Verification items for the finished model (mm, model axes). A direction names the side the tool comes from. Coordinates: 2 decimals unless noted, no trailing zeros. Order: outer loops, then holes, each group sorted by start corner. A loop starts at its lowest first (then second) coordinate and runs counter-clockwise, first axis right, second up.
Q1. Set-up check for faces 1 (the flat face through (-30, -22, -19)), 2 (the cylindrical face through (-7.493, 13.864, 16.826)), 3 (the flat face through (-2, -22, -22)), 4 (the flat face through (-7, 22, 18)): record each of +Z, -Z, +X, -X, +Y, -Y from which the full face is reachable in a straight line by a thin tool's end or side.
Q2. Cross-section at B-B, the plane x = -32. Record the boundary of the cut face in (y, z), and give its area (4 significant figures).
Q3. Thickness scan on line 1 (Y direction, x = -32, z = -23.65); line 2 (Y direction, x = -7.75, z = 20); line 3 (Z direction, x = -41, y = -19.5). Record the ranges inside material, lowest first.
Q4. Cross-section at D-D, the plane x = -13.5. Record the boundary of the cut face in (y, z).
Q5. Draft check along X on faces 5 (the cylindrical face through (-35.966, -10.909, -23.507)), 6 (the flat face through (-10, 22, -10)), 7 (the cylindrical face through (-8, 0, -18)). Enter one of: pulls with the +X half, pulls with the -X half, needs draft (parallel to the pull), parting line crosses it, or undercut.
Q6. Cross-section at C-C, the plane z = -15. Record the boundary of the cut face in (x, y), and give its area (3 significant figures).
Q7. Cross-section at A-A, the plane y = 11.43. Record the boundary of the cut face in (x, z).
Q8. Depth check by flat-ended pin: P1, Ø4, axis at x = -10, z = 4.5, coming from the +Y side; P2, Ø5.5, axis at x = -3.5, y = 13.5, coming from the +Z side; P3, Ø20.5, axis at y = 28.5, z = 10, coming from the -X side; P4, Ø10.5, axis at x = -32, y = -11.43, coming from the -Z side. Enter the tip coordinate at first touch or a pass-through.
Autodesk Inventor part; units mm, degrees
ref_plane "side_2a_XY" through (-32, -21.925, -19) normal (0, 0, 1) x (1, 0, 0)
ref_plane "side_2a_YZ" through (-32, -21.925, -19) normal (1, 0, 0) x (0, 1, 0)
ref_plane "side_2a_ZX" through (-32, -21.925, -19) normal (0, 1, 0) x (0, 0, 1)
sketch "Skizze_34" plane through (0, 0, 0) normal (0, 1, 0) x (1, 0, 0)
  circle A0 centre (0, 12) radius 10
extrude "Extrusion1" add sketch "Skizze_34" along normal mid plane 2.5
sketch "Skizze_35" plane through (0, 0, 0) normal (0, 1, 0) x (1, 0, 0)
  circle A0 centre (0, 12) radius 6
extrude "Extrusion2" add sketch "Skizze_35" along normal mid plane 85.5
sketch "Skizze_36" plane through (0, -1.3, 0) normal (0, 1, 0) x (1, 0, 0)
  line L0 (-50, 24) -> (-50, 21)
  arc A0 (-50, 21) -> (-48, 19) centre (-48, 21) ccw
  line L1 (-48, 19) -> (-12, 19)
  arc A1 (-10, 17) -> (-12, 19) centre (-12, 17) ccw
  line L2 (-10, 17) -> (-10, 12)
  arc A2 (-10, 12) -> (0, 22) centre (0, 12) ccw
  line L3 (0, 22) -> (-4, 22)
  arc A3 (-5.8856, 23.3333) -> (-4, 22) centre (-4, 24) ccw
  arc A4 (-5.8856, 23.3333) -> (-6.8284, 24) centre (-6.8284, 23) ccw
  line L4 (-6.8284, 24) -> (-50, 24)
  circle A5 centre (0, 12) radius 6
extrude "Extrusion3" add sketch "Skizze_36" against normal blind 41.25
sketch "Skizze_37" plane through (0, 1.3, 0) normal (0, 1, 0) x (1, 0, 0)
  line L0 (-12, -38) -> (-9, -38)
  arc A0 (-9, -38) -> (-7, -36) centre (-9, -36) ccw
  line L1 (-7, -36) -> (-7, 0)
  arc A1 (-5, 2) -> (-7, 0) centre (-5, 0) ccw
  line L2 (-5, 2) -> (0, 2)
  arc A2 (0, 2) -> (-10, 12) centre (0, 12) ccw
  line L3 (-10, 12) -> (-10, 8)
  arc A3 (-11.3333, 6.1144) -> (-10, 8) centre (-12, 8) ccw
  arc A4 (-11.3333, 6.1144) -> (-12, 5.1716) centre (-11, 5.1716) ccw
  line L4 (-12, 5.1716) -> (-12, -38)
  circle A5 centre (0, 12) radius 6
extrude "Extrusion4" add sketch "Skizze_37" along normal blind 41.25
sketch "Sketch5" plane through (-12, 1.3, -5.1716) normal (-1, 0, 0) x (0, 0, 1)
  point P0 (25.1716, 10.13)
hole "Drilling 1" at (-12, 11.43, 20) direction (1, 0, 0) diameter 8 depth 5 countersink diameter 16 countersink angle 90
sketch "Sketch6" plane through (-12, 1.3, -5.1716) normal (-1, 0, 0) x (0, 0, 1)
  point P0 (25.1716, 31.13)
hole "Drilling 2" at (-12, 32.43, 20) direction (1, 0, 0) diameter 8 depth 5 countersink diameter 16 countersink angle 90
sketch "Sketch7" plane through (-48, -1.3, -19) normal (0, 0, 1) x (1, 0, 0)
  point P0 (16, -10.13)
hole "Drilling 3" at (-32, -11.43, -19) direction (0, 0, -1) diameter 8 depth 5 countersink diameter 16 countersink angle 90
sketch "Sketch8" plane through (-48, -1.3, -19) normal (0, 0, 1) x (1, 0, 0)
  point P0 (16, -31.13)
hole "Drilling 4" at (-32, -32.43, -19) direction (0, 0, -1) diameter 8 depth 5 countersink diameter 16 countersink angle 90
ref_plane "side_2a_XY" through (-32, -21.925, -19) normal (0, 0, 1) x (1, 0, 0)
ref_plane "side_2a_YZ" through (-32, -21.925, -19) normal (1, 0, 0) x (0, 1, 0)
ref_plane "side_2a_ZX" through (-32, -21.925, -19) normal (0, 1, 0) x (0, 0, 1)
ref_plane "side_2b_XY" through (-32, -21.925, -24) normal (0, 0, -1) x (1, 0, 0)
ref_plane "side_2b_YZ" through (-32, -21.925, -24) normal (1, 0, 0) x (0, -1, 0)
ref_plane "side_2b_ZX" through (-32, -21.925, -24) normal (0, -1, 0) x (0, 0, -1)
ref_plane "side_1b_XY" through (-7, 21.925, 20) normal (1, 0, 0) x (0, 0, -1)
ref_plane "side_1b_YZ" through (-7, 21.925, 20) normal (0, 0, -1) x (0, 1, 0)
ref_plane "side_1b_ZX" through (-7, 21.925, 20) normal (0, 1, 0) x (1, 0, 0)
ref_plane "side_3b_XY" through (-7, 21.925, 20) normal (1, 0, 0) x (0, 0, -1)
ref_plane "side_3b_YZ" through (-7, 21.925, 20) normal (0, 0, -1) x (0, 1, 0)
ref_plane "side_3b_ZX" through (-7, 21.925, 20) normal (0, 1, 0) x (1, 0, 0)
ref_plane "side_1a_XY" through (-12, 21.925, 20) normal (-1, 0, 0) x (0, 0, -1)
ref_plane "side_1a_YZ" through (-12, 21.925, 20) normal (0, 0, -1) x (0, -1, 0)
ref_plane "side_1a_ZX" through (-12, 21.925, 20) normal (0, -1, 0) x (-1, 0, 0)
ref_plane "side_3a_XY" through (-12, 21.925, 20) normal (-1, 0, 0) x (0, 0, -1)
ref_plane "side_3a_YZ" through (-12, 21.925, 20) normal (0, 0, -1) x (0, -1, 0)
ref_plane "side_3a_ZX" through (-12, 21.925, 20) normal (0, -1, 0) x (-1, 0, 0)
properties part number "MayTec 1.62.842032085_Alu hinges, heavy, type 20 PG 40 (90)"
Check values:
1. face 1: +Z, -X, +Y, -Y
1. face 2: +X, -X
1. face 3: -Z, +X, +Y, -Y
1. face 4: +Z, +X, +Y, -Y
2. outline: (-42.55, -24) - (-36.43, -24) - (-36.43, -23) - (-40.43, -19) - (-42.55, -19) - close; (-28.43, -24) - (-15.43, -24) - (-15.43, -23) - (-19.43, -19) - (-24.43, -19) - (-28.43, -23) - close; (-7.43, -24) - (-1.3, -24) - (-1.3, -19) - (-3.43, -19) - (-7.43, -23) - close
2. area: 94.25 mm2
3. line 1: y = -42.55 to -36.43, -28.43 to -15.43, -7.43 to -1.3
3. line 2: y = 1.3 to 7.43, 15.43 to 28.43, 36.43 to 42.55
3. line 3: z = -24 to -19
4. outline: (-42.55, -24) - (-1.3, -24) - (-1.3, -19) - (-42.55, -19) - close
5. face 5: undercut
5. face 6: pulls with the -X half
5. face 7: parting line crosses it
6. outline: (-10, -42.55) - (-5.2, -42.55) - (-5.2, -42.75) - (5.2, -42.75) - (5.2, -42.55) - (9.54, -42.55) - (9.54, -1.3) - (5.2, -1.3) - (5.2, -1.25) - (9.54, -1.25) - (9.54, 1.25) - (5.2, 1.25) - (5.2, 1.3) - (9.54, 1.3) - (9.54, 42.55) - (5.2, 42.55) - (5.2, 42.75) - (-5.2, 42.75) - (-5.2, 42.55) - (-9.54, 42.55) - (-9.54, 1.3) - (-5.2, 1.3) - (-5.2, 1.25) - (-9.54, 1.25) - (-9.54, -1.25) - (-5.2, -1.25) - (-5.2, -1.3) - (-10, -1.3) - close
6. area: 1,650 mm2
7. outline: (-12, -5.17) arc R1 ccw to (-11.33, -6.11) arc R2 cw to (-10, -8) - (-10, -12) arc R10 ccw (long way) to (0, -2) - (-5, -2) arc R2 cw to (-7, 0) - (-7, 16) - (-8, 16) - (-12, 12) - close; (-12, 28) - (-8, 24) - (-7, 24) - (-7, 36) arc R2 ccw to (-9, 38) - (-12, 38) - close
8. P1: stops at y = 42.55
8. P2: stops at z = -1.56
8. P3: stops at x = -12
8. P4: stops at z = -24
